Geometry: see drawing. Coordinates: mm, zero at the bounding-box minimum. Give positions to 0.01 mm unless a question says otherwise; leave off trailing zeros. Loops run counter-clockwise (first coordinate to the right, second up) from the corner with the lowest first, then second, coordinate; pieces in that order, holes last. Notation, with made-up numbers: (-3, -12) -> (36, -12) arc R28 ccw to (36, 13) -> close; hole circle Ø10 at (-29, -1.75). An arc over 180 degrees is marked (long way). Use CSV: the item, a comma, the result in double quotes.
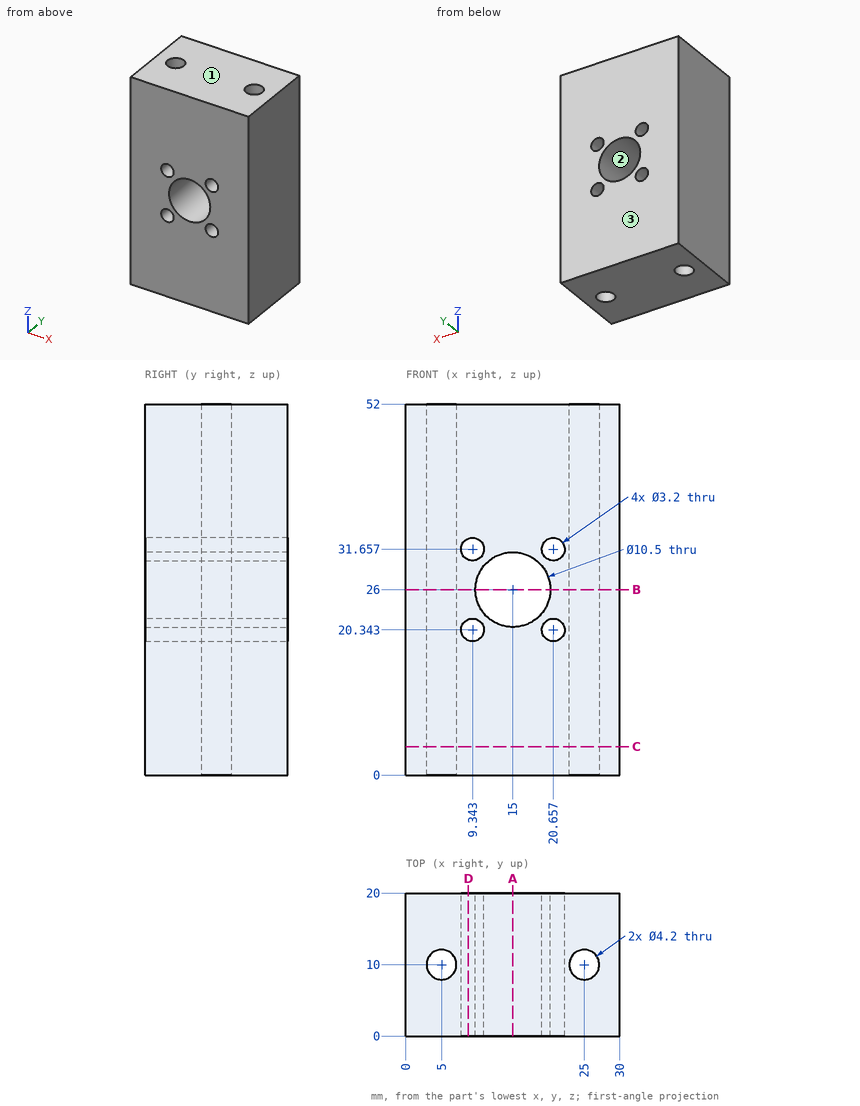
1) Mould query, pull axis Z, two halves, no side actions, for the marked faces 1, 2 and 3. Classes: pulls with the +Z half, pulls with the -Z half, needs draft (parallel to the pull), parting line crosses it, or undercut.
From the geometry:
face 1,"pulls with the +Z half"
face 2,"undercut"
face 3,"needs draft"
2) Section query C-C (z = 4). Return loops of the section in (x, y), then the cut area to 3 significant figures.
From the geometry:
outline,"(0, 0) -> (30, 0) -> (30, 20) -> (0, 20) -> close; hole circle Ø4.2 at (5, 10); hole circle Ø4.2 at (25, 10)"
area,"572 mm^2"
3) Section query A-A (x = 15). Return loops of the section in (y, z).
From the geometry:
outline,"(0, 0) -> (20, 0) -> (20, 20.75) -> (0, 20.75) -> close; (0, 31.25) -> (20, 31.25) -> (20, 52) -> (0, 52) -> close"
4) Section query B-B (z = 26). Return loops of the section in (x, y), then the cut area to 3 significant figures.
From the geometry:
outline,"(0, 0) -> (9.75, 0) -> (9.75, 20) -> (0, 20) -> close; (20.25, 0) -> (30, 0) -> (30, 20) -> (20.25, 20) -> close; hole circle Ø4.2 at (5, 10); hole circle Ø4.2 at (25, 10)"
area,"362 mm^2"
5) Ray query, line 1 (Z direction, x = 9.5, y = 12.75); line 2 (X direction, y = 9.25, z = 15); line 3 (X direction, y = 10, z = 27). Return the intervals inside material, ascending.
From the geometry:
line 1,"z = 0 to 18.75, 21.94 to 30.06, 33.25 to 52"
line 2,"x = 0 to 3.04, 6.96 to 23.04, 26.96 to 30"
line 3,"x = 0 to 2.9, 7.1 to 9.85, 20.15 to 22.9, 27.1 to 30"
6) Contact query for a flat-ended pin moving along its axis: pin 1 (1.9 mm diameter, centred on x = 9.34, z = 31.66, fed in from +Y). Output: stop coordinate, or through.
From the geometry:
pin 1,"passes through"
7) Section query D-D (x = 8.75). Return loops of the section in (y, z).
From the geometry:
outline,"(0, 0) -> (20, 0) -> (20, 18.86) -> (0, 18.86) -> close; (0, 21.83) -> (20, 21.83) -> (20, 30.17) -> (0, 30.17) -> close; (0, 33.14) -> (20, 33.14) -> (20, 52) -> (0, 52) -> close"
